Part model, mm, in its own coordinate system. Face numbers are marked on the shaded views. Give positions to 0.01 mm unless a question says otherwise; leave off trailing zeros. Order: outer loops, then holes, each group sorted by start corner. A loop starts at its lowest first (then second) coordinate and runs counter-clockwise, first axis right, second up. Notation, with made-up numbers: M 58,44 L 68,44 A8 ccw 68,48 Z; hole C -37,67.5 d10. An arc over 180 degrees is marked long. Return JSON: item names as keys, results as strings.
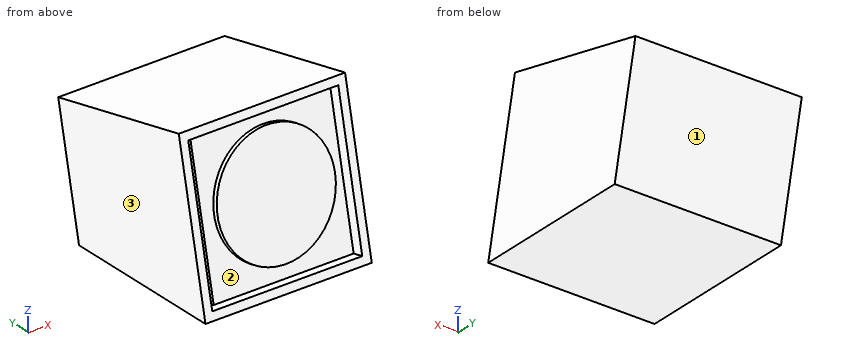
from build123d import *

# Parameters (mm, degrees)
F1_DEPTH = 368.3
F2_W     = 332.232
F2_H     = 319.532
F3_DEPTH = 25.4
F4_R     = 130.175
F5_DEPTH = 10.16
F6_W     = 22.225
F6_H     = 319.532
F7_DEPTH = 50.8


with BuildPart() as f1:
    # F0 (on Right) → F1 (new body)
    with BuildSketch(Plane.YZ):
        Polygon((76.9659267164, 347.1708601318), (0, 0), (364.2337952902, 0), (424.1367868482, 270.2049334155), align=None)
    extrude(amount=F1_DEPTH)

    # F2 (on face) → F3 (cut)
    with BuildSketch(Plane(origin=(0, 0, 0), x_dir=(1, 0, 0), z_dir=(0, -0.9762960071, 0.2164396139))):
        with Locations((184.15, 177.8)):
            Rectangle(F2_W, F2_H)
    extrude(amount=-F3_DEPTH, mode=Mode.SUBTRACT)

    # F4 (on face) → F5 (join)
    with BuildSketch(Plane(origin=(0, 24.7979185808, -5.497566194), x_dir=(1, 0, 0), z_dir=(0, -0.9762960071, 0.2164396139))):
        with Locations((197.866, 177.8)):
            Circle(F4_R)
    extrude(amount=F5_DEPTH)

    # F6 (on face) → F7 (cut)
    with BuildSketch(Plane(origin=(0, 24.7979185808, -5.497566194), x_dir=(1, 0, 0), z_dir=(0, -0.9762960071, 0.2164396139))):
        with Locations((29.1465, 177.8)):
            Rectangle(F6_W, F6_H)
    extrude(amount=-F7_DEPTH, mode=Mode.SUBTRACT)


solid = f1.part
Q1. Band-saw the part on B-B (x = 290.5). Give the cut face in (y, z).
Established:
{"outline": "M 0,0 L 364.23,0 L 424.14,270.2 L 76.97,347.17 L 73.06,329.56 L 97.86,324.07 L 83.08,257.38 L 73.16,259.58 L 33.57,81 L 43.49,78.8 L 28.7,12.11 L 3.9,17.61 Z"}
Q2. Probe line 1 along Z through (x, y) = (284, 302); line 2 along Y through (x, z) = (34, 109); line 3 along Y through (x, z) = (212, 134). List the from-to ranges inside material, lowest first.
Established:
{"line 1": "z = 0 to 297.28", "line 2": "y = 102.21 to 388.4", "line 3": "y = 45.32 to 393.94"}
Q3. Band-saw the part on C-C (y = 216). Give the cut face in (x, z).
Established:
{"outline": "M 0,0 L 368.3,0 L 368.3,316.35 L 0,316.35 Z"}
Q4. Band-saw the part on D-D (x = 135). Give the cut face in (y, z).
Established:
{"outline": "M 0,0 L 364.23,0 L 424.14,270.2 L 76.97,347.17 L 73.06,329.56 L 97.86,324.07 L 87.95,279.37 L 78.03,281.57 L 28.69,59 L 38.61,56.8 L 28.7,12.11 L 3.9,17.61 Z"}
Q5. Band-saw the part on A-A (y = 121.5). Give the cut face in (x, z).
Established:
{"outline": "M 0,0 L 368.3,0 L 368.3,337.3 L 0,337.3 Z; hole M 18.03,195.99 L 40.26,195.99 L 40.26,318.83 L 18.03,318.83 Z"}
Q6. Pin check, flat tips, straight feed: pin 1 (8 mm diameter, centred on x = 222.5, y = 283, fed in from +Z); pin 2 (1 mm diameter, centred on x = 272, z = 239, fed in from -Y); pin 3 (12 mm diameter, centred on x = 258, y = 116.5, fed in from +Z); pin 4 (5 mm diameter, centred on y = 42.5, z = 193.5, fed in from +X). Stop position of each tip, or through.
Established:
{"pin 1": "stops at z = 302.38", "pin 2": "stops at y = 68.48", "pin 3": "stops at z = 339.74", "pin 4": "stops at x = 368.3"}
Q7. Two-plate mould, pull along X, no slides. Class the marked faces 1, 2 and 3: +X half, -X half, draft (parallel to the pull), parting line (faces both ways), or undercut.
Established:
{"face 1": "draft", "face 2": "undercut", "face 3": "-X half"}
